Check sheet for the modelled part. Datum: model origin and axes. Units: mm. A direction names the side the tool comes from. Coordinates: 2 decimals unless noted, no trailing zeros. Order: outer loops, then holes, each group sorted by start corner. A loop starts at its lowest first (then second) coordinate and runs counter-clockwise, first axis right, second up.
1. Set-up check for faces 5 (the flat face through (54.165, 9.03, 8.637)), 6 (the cylindrical face through (44.862, 6.156, 9.889)): record each of +Z, -Z, +X, -X, +Y, -Y from which the full face is reachable in a straight line by a thin tool's end or side.
2. Cross-section at D-D (z = 13.75). Enter the section's corners in (x, y), then the cut area to 3 significant figures.
3. Cross-section at C-C (x = 79). Enter the section's corners in (y, z) (1 decimal).
4. Thickness scan on line 1 (Y direction, x = 68.25, z = 8.76) (3 decimals); line 2 (X direction, y = 13.25, z = 5.5); line 3 (X direction, y = 6.75, z = 6.25). Record the ranges inside material, lowest first.
5. Draft check along Y on faces 1 (the flat face through (35.565, 7.579, 8.637)), 2 (the cylindrical face through (83.888, 8.573, 8.627)), 3 (the flat face through (0, 9, 9)), 4 (the cylindrical face through (73.153, 6.467, 8.487)). Enter one of: released by +Y, released by -Y, zero draft, split by the parting line, or undercut.
6. Cross-section at B-B (y = 8.76). Enter the section's corners in (x, z) (1 decimal).
7. Cross-section at A-A (z = 8.76). Enter the section's corners in (x, y) (1 decimal).
8. Gauge pin test, flat ends, axial feed: pin 1 Ø2 at (x, z) = (56.5, 14) entering from +Y; pin 2 Ø4 at (x, y) = (61.5, 12) entering from -Z; pin 3 Ø3 at (x, y) = (41, 13.5) entering from +Z. Record the tip position at first contact, or that the pin passes through.
```python
from build123d import *

# Parameters (mm, degrees)
BOSS_EXTRUDE3_DEPTH = 17.52
SKETCH5_OUTSIDE_W   = 37.02
SKETCH5_OUTSIDE_H   = 37.174
SKETCH5_OUTSIDE_R   = 8.755
CUT_EXTRUDE7_DEPTH  = 88.487428942
SKETCH6_R           = 2.100334354
CUT_EXTRUDE8_DEPTH  = 88.46999549


with BuildPart() as part:
    # Sketch1 → Boss-Extrude3 (new body)
    with BuildSketch(Plane.XY):
        with BuildLine():
            Line((0, 0), (14.267245849, 0))
            Line((14.267245849, 0), (21.021041326, 14.94364804))
            ThreePointArc((21.021041326, 14.94364804), (26.648105385, 15.66096006), (32.275169445, 14.94364804))
            Line((32.275169445, 14.94364804), (38.949508505, 0))
            Line((38.949508505, 0), (53.219448236, -0.041473561))
            Line((53.219448236, -0.041473561), (54.782126974, 14.94364804))
            ThreePointArc((54.782126974, 14.94364804), (58.376232217, 15.66096006), (61.97033746, 14.94364804))
            Line((61.97033746, 14.94364804), (63.889508505, 0))
            Line((63.889508505, 0), (73.889508505, 0))
            ThreePointArc((73.889508505, 0), (83.889508505, 8.76), (73.889508505, 17.52))
            Line((73.889508505, 17.52), (0, 17.52))
            Line((0, 17.52), (0, 0))
        make_face()
    extrude(amount=BOSS_EXTRUDE3_DEPTH)

    # Sketch5 outside → Cut-Extrude7 (cut, through all)
    with BuildSketch(Plane.ZY):
        with Locations((8.76, 8.76)):
            Rectangle(SKETCH5_OUTSIDE_W, SKETCH5_OUTSIDE_H)
        with Locations((8.76, 8.76)):
            Circle(SKETCH5_OUTSIDE_R, mode=Mode.SUBTRACT)
    extrude(amount=-CUT_EXTRUDE7_DEPTH, mode=Mode.SUBTRACT)

    # Sketch6 → Cut-Extrude8 (cut, through all)
    with BuildSketch(Plane.ZY):
        with Locations((8.76, 4.385)):
            Circle(SKETCH6_R)
    extrude(amount=-CUT_EXTRUDE8_DEPTH, mode=Mode.SUBTRACT)


solid = part.part
```
Data:
1. face 5: +Z, -Z, -Y
1. face 6: +X, -X
2. outline: (0, 1.57) - (14.98, 1.57) - (21.02, 14.94) arc R22.43 cw to (32.28, 14.94) - (38.25, 1.57) - (53.39, 1.57) - (54.78, 14.94) arc R9.36 cw to (61.97, 14.94) - (63.69, 1.57) - (80.18, 1.57) arc R8.84 ccw to (80.18, 15.95) - (0, 15.95) - close
2. area: 834 mm2
3. outline: (0.9, 5) arc R8.8 ccw to (16.7, 5) - (16.7, 12.5) arc R8.8 ccw to (0.9, 12.5) - close; hole circle Ø4.2 at (4.4, 8.8)
4. line 1: y = 0.005 to 2.285, 6.485 to 17.515
4. line 2: x = 0 to 20.26, 33.03 to 54.61, 62.19 to 82.66
4. line 3: x = 0 to 17.32, 35.93 to 53.93, 63.02 to 83.66
5. face 1: released by -Y
5. face 2: split by the parting line
5. face 3: zero draft
5. face 4: undercut
6. outline: (0, 0) - (18.2, 0) - (18.2, 17.5) - (0, 17.5) - close; (35, 0) - (54.1, 0) - (54.1, 17.5) - (35, 17.5) - close; (62.8, 0) - (83.9, 0) - (83.9, 17.5) - (62.8, 17.5) - close
7. outline: (0, 0) - (14.3, 0) - (15.3, 2.3) - (0, 2.3) - close; (0, 6.5) - (17.2, 6.5) - (21, 14.9) arc R22.4 cw to (32.3, 14.9) - (36.1, 6.5) - (53.9, 6.5) - (54.8, 14.9) arc R9.4 cw to (62, 14.9) - (63.1, 6.5) - (83.6, 6.5) arc R8.8 ccw to (76.3, 17.5) - (0, 17.5) - close; (37.9, 2.3) - (38.9, 0) - (53.2, 0) - (53.5, 2.3) - close; (63.6, 2.3) - (63.9, 0) - (76.3, 0) arc R8.8 ccw to (81.1, 2.3) - close
8. pin 1: stops at y = 16.42
8. pin 2: stops at z = 0.14
8. pin 3: stops at z = 16.89
